```python
from build123d import *

# Parameters (mm, degrees)
SKETCH1_W           = 20
SKETCH1_H           = 20
SKETCH1_R           = 9.5
BOSS_EXTRUDE1_DEPTH = 7
FILLET1_R           = 2
SKETCH2_R           = 1.25
CUT_EXTRUDE1_DEPTH  = 16.779733838


with BuildPart() as part:
    # Sketch1 → Boss-Extrude1 (new body)
    with BuildSketch(Plane.XY):
        Rectangle(SKETCH1_W, SKETCH1_H)
        Circle(SKETCH1_R, mode=Mode.SUBTRACT)
    extrude(amount=BOSS_EXTRUDE1_DEPTH)

    # Fillet1
    fillet1_edges = [part.edges().sort_by_distance(p)[0] for p in [
        (10, -10, 3.5),
        (-10, -10, 3.5),
        (-10, 10, 3.5),
        (10, 10, 3.5),
    ]]
    fillet(fillet1_edges, radius=FILLET1_R)

    # Sketch2 → Cut-Extrude1 (cut, through all)
    with BuildSketch(Plane.XY.offset(7)):
        with Locations((-7.825, 7.825)):
            Circle(SKETCH2_R)
        with Locations((7.825, 7.825)):
            Circle(SKETCH2_R)
        with Locations((7.825, -7.825)):
            Circle(SKETCH2_R)
        with Locations((-7.825, -7.825)):
            Circle(SKETCH2_R)
    extrude(amount=-CUT_EXTRUDE1_DEPTH, mode=Mode.SUBTRACT)


solid = part.part
```
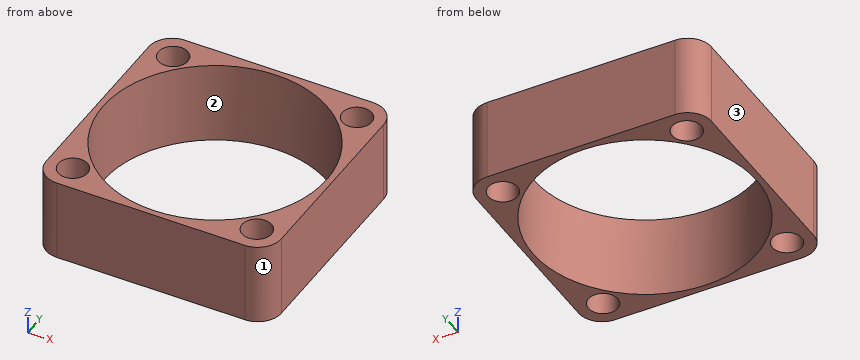
Can you work these out from the model? Positions are in its coordinate system, mm. Face numbers are marked on the shaded views. Coordinates: 2 decimals unless noted, no trailing zeros. Order: outer loops, then holes, each group sorted by start corner. A loop starts at its lowest first (then second) coordinate and runs counter-clockwise, first axis right, second up.
1. If we section it at A-A (y = 0): Please give me the cut outline in (x, z), then the cut area to 3 significant figures.
2. Thinking about a two-plate mould opening in Y: for the marked faces 1, 2 and 3, which applies, +Y half, -Y half, draft (parallel to the pull), parting line (faces both ways), or undercut?
3. I'm going to push a flat-ended pin straight in: pin 1 (3 mm diameter, centred on x = -7.825, y = 7.825, fed in from +Z). Where does the tip first touch, or does it pass through?
4. If we section it at D-D (z = 5): Please give me the cut outline in (x, y) (3 decimals), then the cut area to 3 significant figures.
5. I need wall thicknesses on line 1 (Y direction, x = 0, z = 5.5); line 2 (Y direction, x = 8, z = 3); line 3 (Y direction, x = 8.25, z = 5.75). Which ranges of each line are inside material? Lowest first, please.
6. If we section it at C-C (y = -7): Please give me the cut outline in (x, z), then the cut area to 3 significant figures.
Entries:
1. outline: (-10, 0) - (-9.5, 0) - (-9.5, 7) - (-10, 7) - close; (9.5, 0) - (10, 0) - (10, 7) - (9.5, 7) - close
1. area: 7.00 mm2
2. face 1: -Y half
2. face 2: undercut
2. face 3: draft
3. pin 1: stops at z = 7
4. outline: (-10, -8) arc R2 ccw to (-8, -10) - (8, -10) arc R2 ccw to (10, -8) - (10, 8) arc R2 ccw to (8, 10) - (-8, 10) arc R2 ccw to (-10, 8) - close; hole circle Ø19 at (0, 0); hole circle Ø2.5 at (-7.825, -7.825); hole circle Ø2.5 at (-7.825, 7.825); hole circle Ø2.5 at (7.825, -7.825); hole circle Ø2.5 at (7.825, 7.825)
4. area: 93.4 mm2
5. line 1: y = -10 to -9.5, 9.5 to 10
5. line 2: y = -10 to -9.06, -6.59 to -5.12, 5.12 to 6.59, 9.06 to 10
5. line 3: y = -9.98 to -9, -6.65 to -4.71, 4.71 to 6.65, 9 to 9.98
6. outline: (-10, 0) - (-8.76, 0) - (-8.76, 7) - (-10, 7) - close; (-6.89, 0) - (-6.42, 0) - (-6.42, 7) - (-6.89, 7) - close; (6.42, 0) - (6.89, 0) - (6.89, 7) - (6.42, 7) - close; (8.76, 0) - (10, 0) - (10, 7) - (8.76, 7) - close
6. area: 23.8 mm2
